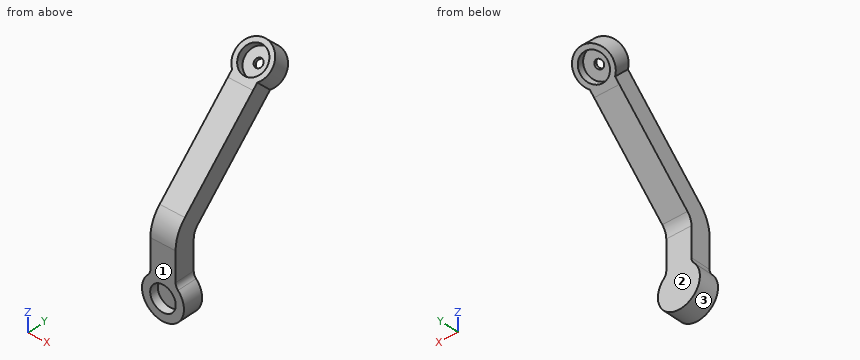
Autodesk Inventor part; units mm, degrees
ref_plane "Work Plane11" through (7.5, -1.606602, 40.312712) normal (0, 0.7071068, -0.7071068) x (-1, 0, 0)
ref_plane "YZ Plane" through (0, 0, 0) normal (1, 0, 0) x (0, 1, 0)
ref_plane "XZ Plane" through (0, 0, 0) normal (0, 1, 0) x (-1, 0, 0)
sketch "Sketch1" plane through (0, 0, 0) normal (0, 1, 0) x (-1, 0, 0)
  arc A0 (-8.928571, 8.748178) -> (8.928571, 8.748178) centre (0, 0) ccw
  line L0 (-7.5, 12.247449) -> (-7.5, 20)
  line L1 (7.5, 20) -> (7.5, 12.247449)
  line L2 (7.5, 20) -> (-7.5, 20)
  arc A1 (7.5, 12.247449) -> (8.928571, 8.748178) centre (12.5, 12.247449) ccw
  arc A2 (-8.928571, 8.748178) -> (-7.5, 12.247449) centre (-12.5, 12.247449) ccw
  point P0 (7.5, 10)
  point P1 (-7.5, 10)
  point P2 (0, 10)
  point P3 (0, 20)
  dimension "d0" = 25
  dimension "d106" = 15
  dimension "d107" = 10
  dimension "d108" = 10
  dimension "d109" = 5
extrude "Extrusion1" add sketch "Sketch1" against normal blind 12
sketch "Sketch22" plane through (-7.5, 0, 20) normal (0, 0, 1) x (1, 0, 0)
  line L0 (0, 0) -> (0, -12)
  line L1 (15, -12) -> (0, -12)
  line L2 (0, 0) -> (15, 0)
  line L3 (15, 0) -> (15, -12)
  line L4 (15, -12) -> (0, -12)
  line L5 (0, -12) -> (0, 0)
  point P0 (7.5, 0)
sketch "Sketch23" plane through (0, 0, 0) normal (1, 0, 0) x (0, 1, 0)
  line L0 (0, 20) -> (-12, 20)
  line L1 (-6, 20) -> (-6, 29.70611)
  line L2 (-1.606602, 40.312712) -> (43.497475, 85.416788)
  arc A0 (-1.606602, 40.312712) -> (-6, 29.70611) centre (9, 29.70611) ccw
  point P0 (0, 0)
  point P1 (-6, 35.919313)
  dimension "d110" = 15.91931
  dimension "d111" = 70
  dimension "d112" = 135
  dimension "d113" = 15
sweep "Sweep2" add profiles "Sketch22" path "Sketch23" path curves L1 A0 L2
ref_plane "Work Plane11" through (7.5, -1.606602, 40.312712) normal (0, 0.7071068, -0.7071068) x (-1, 0, 0)
sketch "Sketch24" plane through (7.5, -1.606602, 40.312712) normal (0, 0.7071068, -0.7071068) x (-1, 0, 0)
  line L0 (0, 63.786797) -> (15, 63.786797)
  line L1 (0, 63.786797) -> (15, 63.786797)
  line L2 (0, 63.786797) -> (0, 67.740058)
  line L3 (15, 63.786797) -> (15, 67.740058)
  arc A0 (15, 67.740058) -> (0, 67.740058) centre (7.5, 75.786797) ccw
  line L4 (0, 63.786797) -> (15, 63.786797)
  point P0 (7.5, -27.369353)
  point P1 (7.5, 63.786797)
  point P2 (7.5, 63.786797)
  dimension "d129" = 22
  dimension "d130" = 12
extrude "Extrusion17" add sketch "Sketch24" along normal mid plane 12
sketch "Sketch25" plane through (-7.5, -5.849242, 44.555352) normal (0, -0.7071068, 0.7071068) x (1, 0, 0)
  circle A0 centre (7.5, 75.786797) radius 2.5
  arc A1 (15, 67.740058) -> (0, 67.740058) centre (7.5, 75.786797) ccw
  point P0 (7.5, -27.369353)
  dimension "d123" = 5
extrude "Extrusion18" cut sketch "Sketch25" against normal through all
sketch "Sketch26" plane through (0, -12, 0) normal (0, -1, 0) x (1, 0, 0)
  circle A0 centre (0, 0) radius 7.6
  dimension "d126" = 15.2
extrude "Extrusion19" cut sketch "Sketch26" against normal blind 5
sketch "Sketch27" plane through (7.5, 2.636039, 36.070071) normal (0, 0.7071068, -0.7071068) x (-1, 0, 0)
  circle A0 centre (7.5, 75.786797) radius 2.5
  circle A1 centre (7.5, 75.786797) radius 8.1
  point P0 (7.5, -27.369353)
  dimension "d131" = 16.2
extrude "Extrusion20" cut sketch "Sketch27" against normal blind 5
mirror "Mirror2" about plane through (7.5, -1.606602, 40.312712) normal (0, 0.7071068, -0.7071068) of "Extrusion20"
properties part number "proximal_link_3"
Work out the finished part from the listing and answer in its coordinate system (mm). Face numbers are marked on the shaded views. Give positions to 0.01 mm unless a question says otherwise; leave off trailing zeros. Order: outer loops, then holes, each group sorted by start corner. A loop starts at its lowest first (then second) coordinate and runs counter-clockwise, first axis right, second up.
1. Straight lines are drawn through the part: L1, parallel to Y at x = -3, z = 12; L2, parallel to Y at x = -1.5, z = 7; L3, parallel to X at y = 23, z = 68. For each, find the intervals that lie inside material, in ascending order.
Result sheet:
L1: y = -12 to 0
L2: y = -7 to 0
L3: x = -7.5 to 7.5
2. Section A-A, the plane z = 0 is taken. Determine the outline of the cut face in (x, y), and give its area (3 significant figures).
Result sheet:
outline: (-12.5, -12) - (-7.6, -12) - (-7.6, -7) - (7.6, -7) - (7.6, -12) - (12.5, -12) - (12.5, 0) - (-12.5, 0) - close
area: 224 mm2
3. The mould has two halves that part along Y. Classify the marked faces 1, 2 and 3: released by +Y, released by -Y, zero draft, split by the parting line, or undercut.
Result sheet:
face 1: released by -Y
face 2: released by +Y
face 3: zero draft
4. Each of these flat-tipped pins is pushed along its axis until it touches: P1, Ø1, axis at x = 3, z = 48.5, coming from the -Y side; P2, Ø7.5, axis at x = 1.5, z = 3, coming from the -Y side; P3, Ø3, axis at x = -1.5, y = 22.5, coming from the -Z side. Where does it stop, or does it pass through?
Result sheet:
P1: stops at y = -2.4
P2: stops at y = -7
P3: stops at z = 54.43
5. Section B-B, the plane x = 0 is taken. Determine the outline of the cut face in (y, z).
Result sheet:
outline: (-12, -12.5) - (0, -12.5) - (0, 29.71) arc R9 cw to (2.64, 36.07) - (50.5, 83.93) - (46.96, 87.47) - (50.92, 91.43) - (49.51, 92.84) - (45.55, 88.88) - (42.01, 92.42) - (-5.85, 44.56) arc R21 ccw to (-12, 29.71) - (-12, 7.6) - (-7, 7.6) - (-7, -7.6) - (-12, -7.6) - close; (53.04, 96.38) - (54.46, 94.96) - (58.42, 98.92) - (61.95, 95.39) - (64, 97.44) - (55.52, 105.92) - (53.47, 103.87) - (57, 100.34) - close
6. Section D-D, the plane z = 14 is taken. Determine the outline of the cut face in (x, y), and give its area (3 significant figures).
Result sheet:
outline: (-7.5, -12) - (7.5, -12) - (7.5, 0) - (-7.5, 0) - close
area: 180 mm2
7. Section C-C, the plane y = 34 is taken. Determine the outline of the cut face in (x, z).
Result sheet:
outline: (-7.5, 67.43) - (7.5, 67.43) - (7.5, 84.4) - (-7.5, 84.4) - close
